Autodesk Inventor part; units mm, degrees
ref_plane "YZ Plane" through (0, 0, 0) normal (1, 0, 0) x (0, 1, 0)
ref_plane "XZ Plane" through (0, 0, 0) normal (0, 1, 0) x (-1, 0, 0)
ref_plane "XY Plane" through (0, 0, 0) normal (0, 0, 1) x (1, 0, 0)
sketch "草圖1" plane through (0, 0, 0) normal (0, 1, 0) x (-1, 0, 0)
  line L0 (-12.5, 5.1777) -> (-5.1777, 12.5)
  line L1 (-5.1777, 12.5) -> (5.1777, 12.5)
  line L2 (5.1777, 12.5) -> (12.5, 5.1777)
  line L3 (12.5, 5.1777) -> (12.5, -5.1777)
  line L4 (12.5, -5.1777) -> (5.1777, -12.5)
  line L5 (5.1777, -12.5) -> (-5.1777, -12.5)
  line L6 (-5.1777, -12.5) -> (-12.5, -5.1777)
  line L7 (-12.5, -5.1777) -> (-12.5, 5.1777)
  line L8 (123.9504, 0) -> (-90.7739, 0) construction
  point P0 (0, 0)
  point P1 (0, 0)
  dimension "d1" = 25
extrude "擠出1" add sketch "草圖1" along normal blind 12
shell "薄殼3" thickness 5 removed faces 1 at (-0.7149, 12, -1.7259) ; own thickness 5 on faces at (1.7259, 4, 12.5) (10.0592, 4, 7.6184) ; own thickness 3 on faces at (12.5, 4, -1.7259) ; own thickness 1 on faces at (-7.6184, 4, 10.0592) (-12.5, 4, 1.7259) (-10.0592, 4, -7.6184) (-1.7259, 4, -12.5) (7.6184, 4, -10.0592)
properties part number "示範一"
Verification items for the finished model (mm, model axes). A direction names the side the tool comes from. Coordinates: 2 decimals unless noted, no trailing zeros. Loops run counter-clockwise (first coordinate to the right, second up) from the corner with the lowest first, then second, coordinate; pieces in that order, holes last. Notation, with made-up numbers: (44, 34) -> (87, 34) arc R11 cw to (87, 44) -> close; hole circle Ø3 at (82.25, 64.5). An arc over 180 degrees is marked (long way). Answer as a JSON object with one key per item and string values. Group by question number.
Item 1: Sectioned sample at D-D on z = 10.5. Record the boundary of the cut face in (x, y), plus the area to 3 significant figures.
Item 2: Sectioned sample at A-A on y = 11. Record the boundary of the cut face in (x, z).
Item 3: Scan lines: probe 1 along Z at (x, y) = (-4, 9.5); probe 2 along X at (y, z) = (7.5, -3); probe 3 along Y at (x, z) = (-6.5, 0.25). Record each from-to range of solid material in increasing order.
Item 4: Sectioned sample at C-C on x = 2. Record the boundary of the cut face in (y, z), plus the area to 3 significant figures.
Item 5: Depth check by flat-ended pin: pin 1 (2 mm diameter, centred on x = -6, z = -8, fed in from +Y); pin 2 (6 mm diameter, centred on x = -8.5, y = 8.5, fed in from +Z); pin 3 (6 mm diameter, centred on y = 7, z = -9, fed in from +X). Enter the tip coordinate at first touch or a pass-through.
Item 6: Mould release check, pull along X, two halves, no side actions. Record for faces 1 (the flat face through (-3, 8, 7.5)), 2 (the flat face through (12.5, 6, 0)), 3 (the flat face through (0, 6, 12.5)): +X half, -X half, draft (parallel to the pull), parting line (faces both ways), or undercut.
Item 7: Tool access check on faces 4 (the flat face through (7.099, 8.451, -9.165)), 5 (the flat face through (-12.5, 6, 0)). Record the directions out of +Z, -Z, +X, -X, +Y, -Y that give a thin tool (end or side, any length) a straight path to the whole face; none if there is none.
Item 8: Sectioned sample at B-B on z = -1.5. Record the boundary of the cut face in (x, y), plus the area to 3 significant figures.
Evaluation:
{
 "1": {"outline": "(-7.18, 0) -> (7.18, 0) -> (7.18, 12) -> (-7.18, 12) -> close", "area": "172 mm²"},
 "2": {"outline": "(-12.5, -5.18) -> (-5.18, -12.5) -> (5.18, -12.5) -> (12.5, -5.18) -> (12.5, 5.18) -> (5.18, 12.5) -> (-5.18, 12.5) -> (-12.5, 5.18) -> close; hole (-11.5, -4.76) -> (-4.76, -11.5) -> (4.76, -11.5) -> (9.5, -6.76) -> (9.5, 1.11) -> (3.11, 7.5) -> (-8.76, 7.5) -> (-11.5, 4.76) -> close"},
 "3": {"probe 1": "z = -12.5 to -11.5, 7.5 to 12.5", "probe 2": "x = -12.5 to -11.5, 9.5 to 12.5", "probe 3": "y = 0 to 5"},
 "4": {"outline": "(0, -12.5) -> (12, -12.5) -> (12, -11.5) -> (5, -11.5) -> (5, 7.5) -> (12, 7.5) -> (12, 12.5) -> (0, 12.5) -> close", "area": "167 mm²"},
 "5": {"pin 1": "stops at y = 5", "pin 2": "stops at z = 12.18", "pin 3": "stops at x = 11.68"},
 "6": {"face 1": "undercut", "face 2": "+X half", "face 3": "draft"},
 "7": {"face 4": "+Y", "face 5": "+Z, -Z, -X, +Y, -Y"},
 "8": {"outline": "(-12.5, 0) -> (12.5, 0) -> (12.5, 12) -> (9.5, 12) -> (9.5, 5) -> (-11.5, 5) -> (-11.5, 12) -> (-12.5, 12) -> close", "area": "153 mm²"}
}
